Answer from the drawing. Dimensions are ordinates in mm from the lowest x, y and z of the part. A direction names the side the tool comes from. Give positions to 0.01 mm unless a question says otherwise; leave off trailing zeros. Loops run counter-clockwise (first coordinate to the right, second up) from the corner with the lowest first, then second, coordinate; pieces in that order, holes last.
(1) Straight lines are drawn through the part: probe 1 along Y at (x, z) = (21.5, 112.5); probe 2 along X at (y, z) = (18.5, 90). For each, find the intervals that lie inside material, in ascending order.
(2) This flat-tipped pin is pushed along its axis until it touches: P1, Ø1.5, axis at x = 30.5, z = 17.5, coming from the -Y side. Where does it stop, or does it pass through?
(3) Which of the six approach directions +Z, -Z, +X, -X, +Y, -Y give full straight-line access (tool end or side, diameter ignored) to the marked faces 1 and 2?
(4) Find section C-C, the plane x = 24. Write down the section's boundary in (y, z).
(5) Determine the mould class of the marked faces 3, 4 and 5 for opening direction X: pulls with the +X half, pulls with the -X half, needs draft (parallel to the pull), parting line crosses it, or undercut.
(6) Find section A-A, the plane y = 75. Write down the section's boundary in (x, z).
(7) Find section B-B, the plane z = 52.5. Write down the section's boundary in (x, y).
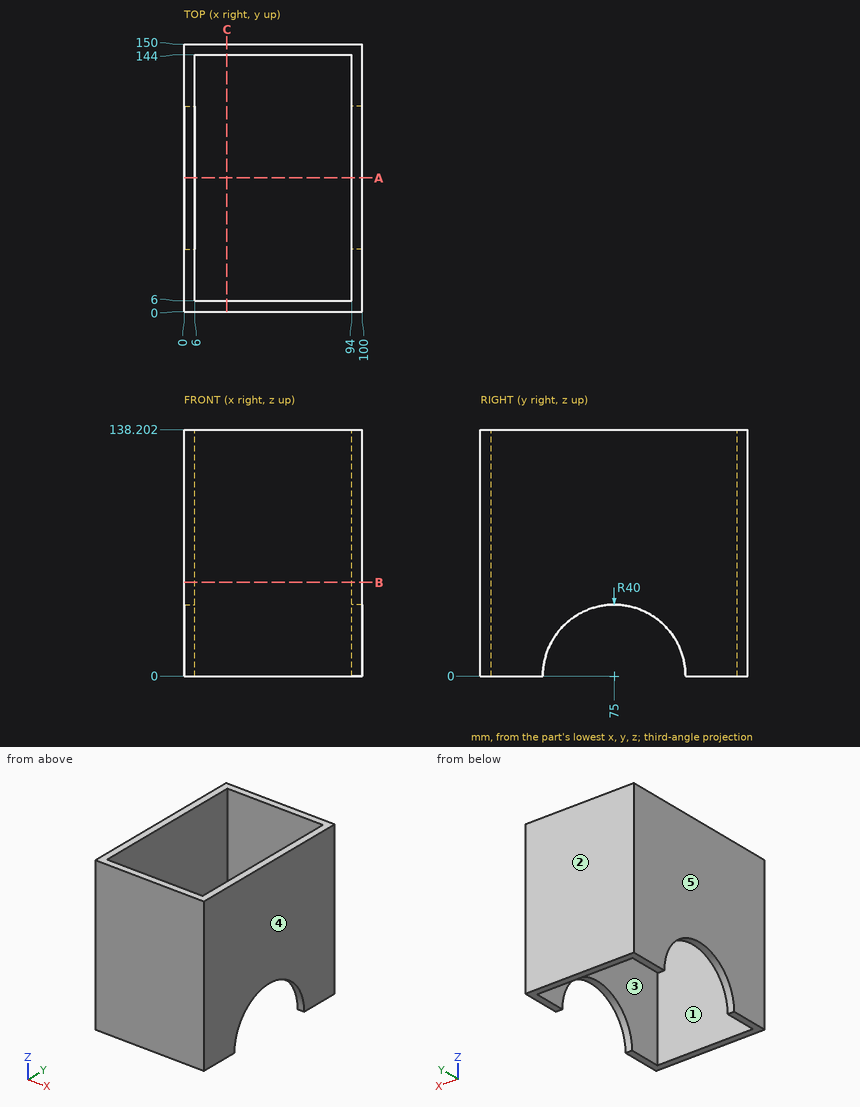
Entries:
1. probe 1: y = 0 to 6, 144 to 150
1. probe 2: x = 0 to 6, 94 to 100
2. P1: stops at y = 0
3. face 1: +Z, -Z
3. face 2: +Z, -Z, +X, -X, +Y
4. outline: (0, 0) - (6, 0) - (6, 138.2) - (0, 138.2) - close; (144, 0) - (150, 0) - (150, 138.2) - (144, 138.2) - close
5. face 3: undercut
5. face 4: pulls with the +X half
5. face 5: pulls with the -X half
6. outline: (0, 40) - (6, 40) - (6, 138.2) - (0, 138.2) - close; (94, 40) - (100, 40) - (100, 138.2) - (94, 138.2) - close
7. outline: (0, 0) - (100, 0) - (100, 150) - (0, 150) - close; hole (6, 6) - (94, 6) - (94, 144) - (6, 144) - close
